from build123d import *

# Parameters (mm, degrees)
BOSS_EXTRUDE1_DEPTH = 2
SKETCH2_W           = 49
SKETCH2_H           = 2
BOSS_EXTRUDE2_DEPTH = 8
SKETCH3_R           = 0.8
CUT_EXTRUDE1_DEPTH  = 2
SKETCH4_R           = 0.8
CUT_EXTRUDE2_DEPTH  = 2
CUT_EXTRUDE3_DEPTH  = 2


with BuildPart() as part:
    # Sketch1 → Boss-Extrude1 (new body)
    with BuildSketch(Plane.XY):
        Polygon((42.5, 17), (49, 17), (49, 0), (0, 0), (0, 17), (6.5, 17), (6.5, 2), (42.5, 2), align=None)
    extrude(amount=BOSS_EXTRUDE1_DEPTH)

    # Sketch2 → Boss-Extrude2 (add)
    with BuildSketch(Plane.XY.offset(2)):
        with Locations((24.5, 1)):
            Rectangle(SKETCH2_W, SKETCH2_H)
    extrude(amount=BOSS_EXTRUDE2_DEPTH)

    # Sketch3 → Cut-Extrude1 (cut)
    with BuildSketch(Plane.XY.offset(2)):
        with Locations((3.25, 13)):
            Circle(SKETCH3_R)
        with Locations((3.25, 6)):
            Circle(SKETCH3_R)
        with Locations((45.75, 13)):
            Circle(SKETCH3_R)
        with Locations((45.75, 6)):
            Circle(SKETCH3_R)
    extrude(amount=-CUT_EXTRUDE1_DEPTH, mode=Mode.SUBTRACT)

    # Sketch4 → Cut-Extrude2 (cut)
    with BuildSketch(Plane(origin=(0, 2, 0), x_dir=(1, 0, 0), z_dir=(0, 1, 0))):
        with Locations(Location((3, -6, 0), (0, 0, 270))):
            Circle(SKETCH4_R)
        with Locations(Location((46, -6, 0), (0, 0, 270))):
            Circle(SKETCH4_R)
    extrude(amount=-CUT_EXTRUDE2_DEPTH, mode=Mode.SUBTRACT)

    # Sketch5 → Cut-Extrude3 (cut)
    with BuildSketch(Plane(origin=(0, 2, 0), x_dir=(1, 0, 0), z_dir=(0, 1, 0))):
        with BuildLine():
            Line((6.5, -10), (6.5, -9))
            ThreePointArc((6.5, -9), (7.964466094, -5.464466094), (11.5, -4))
            Line((11.5, -4), (37.5, -4))
            ThreePointArc((37.5, -4), (41.035533906, -5.464466094), (42.5, -9))
            Line((42.5, -9), (42.5, -10))
            Line((42.5, -10), (6.5, -10))
        make_face()
    extrude(amount=-CUT_EXTRUDE3_DEPTH, mode=Mode.SUBTRACT)


solid = part.part
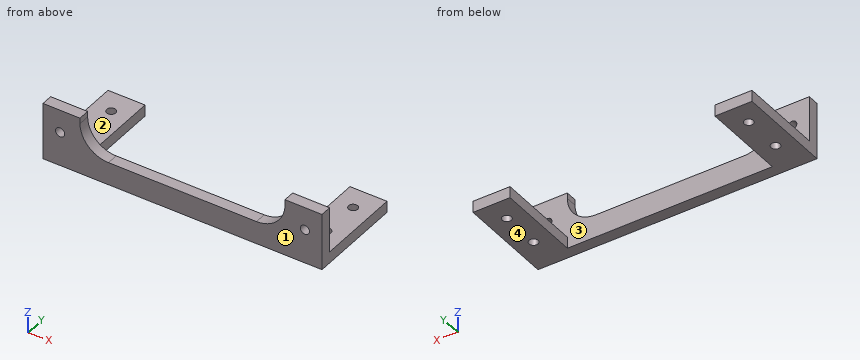
The listing builds one solid part. Answer for the finished solid, in the listing's coordinates (mm). Face numbers are marked on the shaded views. A direction names the side the tool comes from. Round coordinates to 2 decimals unless told otherwise and drop trailing zeros. Write each loop counter-clockwise with the first axis right and the second up, starting at its lowest first coordinate (ties: lowest second). Pieces come first, ordered by that corner, then holes. Notation, with made-up numbers: (39, -40) - (46, -40) arc R24 cw to (46, -3) - close; hole circle Ø2 at (21.25, 89). An arc over 180 degrees is marked (long way). Use a Markdown table: item, result. Add a question column.
1. The part is cut by section C-C (z = 8.25). Write down the section's boundary in (x, y), and give its area (3 significant figures).
2. The part is cut by section D-D (y = 13). Write down the section's boundary in (x, z).
3. The part is cut by section A-A (y = 8.25). Write down the section's boundary in (x, z).
4. Consider line 1 (Y direction, x = 3.25, z = 0.65); line 2 (Z direction, x = 46, y = 0.85); line 3 (X direction, y = 0.85, z = 6). Determine where each line is inside the solid, lowest interval first.
5. Flat-ended cylindrical pins translate along their axes: P1, Ø3, axis at x = 47, y = 9.5, coming from the +Z side; P2, Ø1.4, axis at x = 45.75, y = 6, coming from the -Z side; P3, Ø4, axis at x = 9.5, z = 3.5, coming from the +Y side; P4, Ø1.6, axis at x = 29.5, y = 1.5, coming from the +Z side. Find the tip coordinate at first contact, or state that the pin passes through.
6. For a pull along X with two mould halves and no side action, classify the marked faces 3 and 4 as +X half, -X half, draft (parallel to the pull), parting line (faces both ways), or undercut.
7. The part is cut by section B-B (z = 0.75). Write down the section's boundary in (x, y), and give its area (3 significant figures).
8. A tool of negligible diameter and unlimited length cuts with its end or side. For the marked faces 1 and 2, from which of +Z, -Z, +X, -X, +Y, -Y can it reach the whole face along a straight path? Write none if from no direction.
Reported:
| question | item | result |
|---|---|---|
| 1 | outline | (0, 0) - (6.56, 0) - (6.56, 2) - (0, 2) - close; (42.44, 0) - (49, 0) - (49, 2) - (42.44, 2) - close |
| 1 | area | 26.2 mm^2 |
| 2 | outline | (0, 0) - (2.45, 0) - (2.45, 2) - (0, 2) - close; (4.05, 0) - (6.5, 0) - (6.5, 2) - (4.05, 2) - close; (42.5, 0) - (44.95, 0) - (44.95, 2) - (42.5, 2) - close; (46.55, 0) - (49, 0) - (49, 2) - (46.55, 2) - close |
| 3 | outline | (0, 0) - (6.5, 0) - (6.5, 2) - (0, 2) - close; (42.5, 0) - (49, 0) - (49, 2) - (42.5, 2) - close |
| 4 | line 1 | 0 to 5.2, 6.8 to 12.2, 13.8 to 17 |
| 4 | line 2 | 0 to 5.2, 6.8 to 10 |
| 4 | line 3 | 0 to 2.2, 3.8 to 7.5, 41.5 to 45.2, 46.8 to 49 |
| 5 | P1 | z = 2 |
| 5 | P2 | through |
| 5 | P3 | y = 2 |
| 5 | P4 | z = 4 |
| 6 | face 3 | undercut |
| 6 | face 4 | draft |
| 7 | outline | (0, 0) - (49, 0) - (49, 17) - (42.5, 17) - (42.5, 2) - (6.5, 2) - (6.5, 17) - (0, 17) - close; hole circle Ø1.6 at (3.25, 6); hole circle Ø1.6 at (3.25, 13); hole circle Ø1.6 at (45.75, 6); hole circle Ø1.6 at (45.75, 13) |
| 7 | area | 285 mm^2 |
| 8 | face 1 | +Z, -Z, +X, -X, -Y |
| 8 | face 2 | +Z, +X, -X, +Y |
